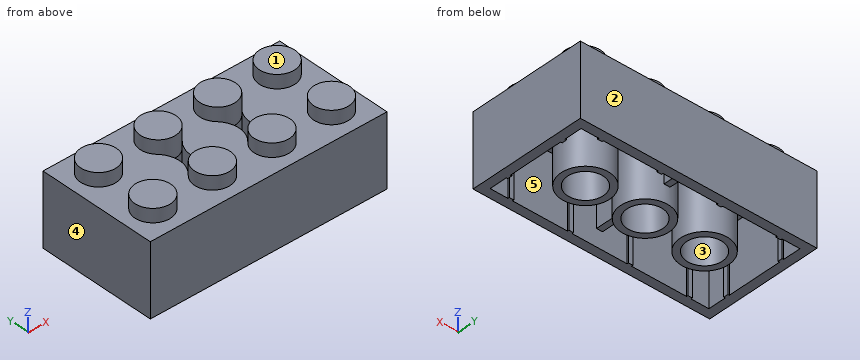
Autodesk Fusion 360 part; units mm, degrees
sketch "side" plane through (0, 0, 0) normal (1, 0, 0) x (0, 1, 0)
  line L0 (0, 0) -> (15.8, 0)
  line L1 (15.8, 0) -> (15.8, 9.6)
  line L2 (15.8, 9.6) -> (0, 9.6)
  line L3 (0, 9.6) -> (0, 0)
  dimension "d1" = 15.8
  dimension "d2" = 9.6
sketch "top" plane through (0, 0, 0) normal (0, 0, 1) x (1, 0, 0)
  line L0 (0, 0) -> (-31.8, 0)
  line L1 (-31.8, 0) -> (-31.8, 15.8)
  line L2 (-31.8, 15.8) -> (0, 15.8)
  line L3 (0, 15.8) -> (0, 0)
  circle A0 centre (-3.9, 11.9) radius 2.4
  line L4 (0, 15.8) -> (0, 0)
  circle A1 centre (-11.9, 11.9) radius 2.4
  circle A2 centre (-19.9, 11.9) radius 2.4
  circle A3 centre (-27.9, 11.9) radius 2.4
  circle A4 centre (-3.9, 3.9) radius 2.4
  circle A5 centre (-11.9, 3.9) radius 2.4
  circle A6 centre (-19.9, 3.9) radius 2.4
  circle A7 centre (-27.9, 3.9) radius 2.4
  circle A8 centre (-7.9, 7.9) radius 3.255
  circle A9 centre (-7.9, 7.9) radius 2.4
  circle A10 centre (-3.9, 11.9) radius 1.3
  circle A11 centre (-3.9, 3.9) radius 1.3
  circle A12 centre (-11.9, 11.9) radius 1.3
  circle A13 centre (-11.9, 3.9) radius 1.3
  circle A14 centre (-19.9, 11.9) radius 1.3
  circle A15 centre (-19.9, 3.9) radius 1.3
  circle A16 centre (-27.9, 11.9) radius 1.3
  circle A17 centre (-27.9, 3.9) radius 1.3
  circle A18 centre (-15.9, 7.9) radius 3.255
  circle A19 centre (-23.9, 7.9) radius 3.255
  circle A20 centre (-15.9, 7.9) radius 2.4
  circle A21 centre (-23.9, 7.9) radius 2.4
  line L5 (-30.6, 14.6) -> (-1.2, 14.6)
  line L6 (-1.2, 14.6) -> (-1.2, 1.2)
  line L7 (-1.2, 1.2) -> (-30.6, 1.2)
  line L8 (-30.6, 1.2) -> (-30.6, 14.6)
  line L9 (-15.9, 7.9) -> (-15.9, 14.6) construction
  line L10 (-15.9, 7.9) -> (-15.9, 1.2) construction
  line L11 (-16.3, 11.1303) -> (-16.3, 14.6)
  line L12 (-15.5, 11.1303) -> (-15.5, 14.6)
  line L13 (-15.5, 4.6697) -> (-15.5, 1.2)
  line L14 (-16.3, 4.6697) -> (-16.3, 1.2)
  line L15 (-28.2, 14.6) -> (-27.6, 14.6)
  line L16 (-27.6, 14.6) -> (-27.6, 14.4)
  line L17 (-27.6, 14.4) -> (-28.2, 14.4)
  line L18 (-28.2, 14.4) -> (-28.2, 14.6)
  line L19 (-20.2, 14.6) -> (-19.6, 14.6)
  line L20 (-19.6, 14.6) -> (-19.6, 14.4)
  line L21 (-19.6, 14.4) -> (-20.2, 14.4)
  line L22 (-20.2, 14.4) -> (-20.2, 14.6)
  line L23 (-12.2, 14.6) -> (-11.6, 14.6)
  line L24 (-11.6, 14.6) -> (-11.6, 14.4)
  line L25 (-11.6, 14.4) -> (-12.2, 14.4)
  line L26 (-12.2, 14.4) -> (-12.2, 14.6)
  line L27 (-4.2, 14.4) -> (-3.6, 14.4)
  line L28 (-3.6, 14.4) -> (-3.6, 14.6)
  line L29 (-3.6, 14.6) -> (-4.2, 14.6)
  line L30 (-4.2, 14.6) -> (-4.2, 14.4)
  line L31 (-1.4, 12.2) -> (-1.2, 12.2)
  line L32 (-1.2, 12.2) -> (-1.2, 11.6)
  line L33 (-1.2, 11.6) -> (-1.4, 11.6)
  line L34 (-1.4, 11.6) -> (-1.4, 12.2)
  line L35 (-1.4, 4.2) -> (-1.2, 4.2)
  line L36 (-1.2, 4.2) -> (-1.2, 3.6)
  line L37 (-1.2, 3.6) -> (-1.4, 3.6)
  line L38 (-1.4, 3.6) -> (-1.4, 4.2)
  line L39 (-4.2, 1.4) -> (-3.6, 1.4)
  line L40 (-3.6, 1.4) -> (-3.6, 1.2)
  line L41 (-3.6, 1.2) -> (-4.2, 1.2)
  line L42 (-4.2, 1.2) -> (-4.2, 1.4)
  line L43 (-11.6, 1.4) -> (-12.2, 1.4)
  line L44 (-12.2, 1.4) -> (-12.2, 1.2)
  line L45 (-12.2, 1.2) -> (-11.6, 1.2)
  line L46 (-11.6, 1.2) -> (-11.6, 1.4)
  line L47 (-19.6, 1.4) -> (-20.2, 1.4)
  line L48 (-20.2, 1.4) -> (-20.2, 1.2)
  line L49 (-20.2, 1.2) -> (-19.6, 1.2)
  line L50 (-19.6, 1.2) -> (-19.6, 1.4)
  line L51 (-27.6, 1.4) -> (-28.2, 1.4)
  line L52 (-28.2, 1.4) -> (-28.2, 1.2)
  line L53 (-28.2, 1.2) -> (-27.6, 1.2)
  line L54 (-27.6, 1.2) -> (-27.6, 1.4)
  line L55 (-30.4, 4.2) -> (-30.6, 4.2)
  line L56 (-30.6, 4.2) -> (-30.6, 3.6)
  line L57 (-30.6, 3.6) -> (-30.4, 3.6)
  line L58 (-30.4, 3.6) -> (-30.4, 4.2)
  line L59 (-30.4, 12.2) -> (-30.6, 12.2)
  line L60 (-30.6, 12.2) -> (-30.6, 11.6)
  line L61 (-30.6, 11.6) -> (-30.4, 11.6)
  line L62 (-30.4, 11.6) -> (-30.4, 12.2)
  dimension "d3" = 31.8
  dimension "d4" = 15.8
  dimension "d5" = 4.8
  dimension "d6" = 3.9
  dimension "d7" = 3.9
  dimension "d8" = 4.8
  dimension "d9" = 4.8
  dimension "d10" = 4.8
  dimension "d11" = 4.8
  dimension "d12" = 4.8
  dimension "d13" = 4.8
  dimension "d14" = 4.8
  dimension "d15" = 3.9
  dimension "d16" = 3.9
  dimension "d17" = 3.9
  dimension "d18" = 8
  dimension "d19" = 8
  dimension "d20" = 8
  dimension "d21" = 8
  dimension "d22" = 8
  dimension "d23" = 8
  dimension "d24" = 3.9
  dimension "d25" = 8
  dimension "d26" = 8
  dimension "d27" = 8
  dimension "d28" = 8
  dimension "d29" = 6.51
  dimension "d30" = 7.9
  dimension "d31" = 7.9
  dimension "d32" = 4.8
  dimension "d33" = 2.6
  dimension "d34" = 2.6
  dimension "d35" = 2.6
  dimension "d36" = 2.6
  dimension "d37" = 2.6
  dimension "d38" = 2.6
  dimension "d39" = 2.6
  dimension "d40" = 2.6
  dimension "d41" = 6.51
  dimension "d42" = 6.51
  dimension "d43" = 8
  dimension "d44" = 7.9
  dimension "d45" = 8
  dimension "d46" = 7.9
  dimension "d47" = 4.8
  dimension "d48" = 4.8
  dimension "d49" = 1.2
  dimension "d50" = 1.2
  dimension "d51" = 1.2
  dimension "d52" = 1.2
  dimension "d53" = 0.8
  dimension "d54" = 0.4
  dimension "d55" = 0.4
  dimension "d56" = 0.8
  dimension "d57" = 0.6
  dimension "d58" = 0.2
  dimension "d60" = 0.6
  dimension "d61" = 0.3
  dimension "d62" = 0.6
  dimension "d63" = 0.3
  dimension "d64" = 0.6
  dimension "d65" = 0.3
  dimension "d66" = 0.6
  dimension "d67" = 0.3
  dimension "d68" = 0.6
  dimension "d69" = 0.6
  dimension "d70" = 0.6
  dimension "d71" = 0.6
  dimension "d72" = 0.6
  dimension "d73" = 0.6
  dimension "d74" = 0.3
  dimension "d75" = 0.6
extrude "Extrude1" add sketch "top" along normal blind 9.6 contours L0 L1 L2 L3 L4 | L5 L23 L24 L25 L26 | L5 L19 L20 L21 L22 | L7 L43 L44 L45 L46 | L5 L27 L28 L29 L30 | L7 L47 L48 L49 L50 | L5 L15 L16 L17 L18 | L7 L39 L40 L41 L42 | L7 L51 L52 L53 L54 | L6 L31 L32 L33 L34 | L8 L59 L60 L61 L62 | L6 L35 L36 L37 L38 | L8 L55 L56 L57 L58 makes body 1
extrude "Extrude2" add sketch "top" along normal blind 9.6 and the other way blind -8.6 contours A0 | A4 | A1 A5 A8 A18 L5 L6 L7 L12 L13 L24 L25 L26 L27 L28 L30 L31 L33 L34 L35 L37 L38 L39 L40 L42 L43 L44 L46 | A8 | A1 | A18 | A5 | A18 L5 L11 L12 | A7 | A3 | A2 A6 A18 A19 L5 L7 L8 L11 L14 L16 L17 L18 L20 L21 L22 L47 L48 L50 L51 L52 L54 L55 L57 L58 L59 L61 L62 | A18 L7 L13 L14 | A2 | A19 | A6 | A9 | A20 | A21 bodies 1
extrude "Extrude3" add sketch "top" along normal blind 9.6 and the other way blind -11.4 contours A0 | A4 | A1 | A5 | A7 | A3 | A2 | A6 | A10 | A11 | A12 | A13 | A14 | A15 | A16 | A17 bodies 1
extrude "Extrude4" cut sketch "top" along normal blind 10.3 and the other way blind -9.6 contours A10 | A11 | A12 | A13 | A14 | A15 | A16 | A17 bodies 1
extrude "Extrude5" add sketch "top" along normal blind 8.6 contours A8 | A18 | A19 bodies 1
extrude "Extrude6" add sketch "top" along normal blind 8.6 and the other way blind -2.3 contours A18 L5 L11 L12 | A18 L7 L13 L14 bodies 1
copy_body "Body->Comp1" bodies 1 removing the originals makes body 2 in component "Piesa Lego 4x2"
component "Piesa Lego 4x2" placed x (1, 0, 0) y (0, 1, 0) z (0, 0, 1) at (0, 0, 0)
equation "d84 = -9.6 mm - 1.8 mm"
equation "d86 = 8.60 mm + 1.7 mm"
For this review, take the finished solid that the model builds, in its own axes (mm). Face numbers are marked on the shaded views. A direction names the side the tool comes from. Round coordinates to 2 decimals unless told otherwise and drop trailing zeros. Order: outer loops, then holes, each group sorted by start corner. A loop starts at its lowest first (then second) coordinate and runs counter-clockwise, first axis right, second up. Notation, with made-up numbers: (81, 30) -> (124, 30) arc R9 cw to (124, 43) -> close; hole circle Ø6 at (49, 46.5). An arc over 180 degrees is marked (long way). Use a Markdown table: item, result.
Item 1: Draft analysis for pull direction Y (two halves, no side actions). For the marked faces 1, 2 and 3, state which applies: +Y half, -Y half, draft (parallel to the pull), parting line (faces both ways), or undercut.
Resolved:
| item | result |
|---|---|
| face 1 | draft |
| face 2 | +Y half |
| face 3 | undercut |
Item 2: For pin 1 (4 mm diameter, centred on x = -3.9, y = 11.9, fed in from -Z), flat-tipped, find the tip position at first contact; note if it passes through.
Resolved:
| item | result |
|---|---|
| pin 1 | stops at z = 8.6 |
Item 3: Take a section at D-D (z = 4.5). State how many separate pieces and enclosed holes the cut face has, plus the area to 3 significant figures.
Resolved:
| item | result |
|---|---|
| separate pieces | 3 |
| enclosed holes | 5 |
| area | 161 mm² |
Item 4: For line 1 along X through (y, z) = (1.5, 7.25); line 2 along Y through (x, z) = (-23.9, 2.5) (3 decimals); line 3 along X through (y, z) = (4, 6.25), list the stretches that pass through material, from the lowest coordinate up. Write a range as [from, to].
Resolved:
| item | result |
|---|---|
| line 1 | x = [-31.8, -30.6], [-16.3, -15.5], [-1.2, 0] |
| line 2 | y = [0, 1.2], [4.645, 5.5], [10.3, 11.155], [14.6, 15.8] |
| line 3 | x = [-31.8, -30.4], [-16.3, -15.5], [-1.4, 0] |
Item 5: Take a section at A-A (x = -11.9). State the section outline as (y, z) points, plus the area to 3 significant figures.
Resolved:
| item | result |
|---|---|
| outline | (0, 0) -> (1.4, 0) -> (1.4, 8.6) -> (2.6, 8.6) -> (2.6, 10.3) -> (5.2, 10.3) -> (5.2, 8.6) -> (6.3, 8.6) -> (6.3, 11.4) -> (1.5, 11.4) -> (1.5, 9.6) -> (0, 9.6) -> close; (9.5, 8.6) -> (10.6, 8.6) -> (10.6, 10.3) -> (13.2, 10.3) -> (13.2, 8.6) -> (14.4, 8.6) -> (14.4, 0) -> (15.8, 0) -> (15.8, 9.6) -> (14.3, 9.6) -> (14.3, 11.4) -> (9.5, 11.4) -> close |
| area | 45.1 mm² |
Item 6: Take a section at B-B (x = -27.9). State the section outline as (y, z) points, plus the area to 3 significant figures.
Resolved:
| item | result |
|---|---|
| outline | (0, 0) -> (1.4, 0) -> (1.4, 8.6) -> (2.6, 8.6) -> (2.6, 10.3) -> (5.2, 10.3) -> (5.2, 8.6) -> (10.6, 8.6) -> (10.6, 10.3) -> (13.2, 10.3) -> (13.2, 8.6) -> (14.4, 8.6) -> (14.4, 0) -> (15.8, 0) -> (15.8, 9.6) -> (14.3, 9.6) -> (14.3, 11.4) -> (9.5, 11.4) -> (9.5, 9.6) -> (6.3, 9.6) -> (6.3, 11.4) -> (1.5, 11.4) -> (1.5, 9.6) -> (0, 9.6) -> close |
| area | 48.3 mm² |
Item 7: Machinability: for the marked faces 4 and 5, which of the approach directions +Z, -Z, +X, -X, +Y, -Y give a long, thin tool a straight path to every point of the face, cutting with its end or side? Answer none if there is none.
Resolved:
| item | result |
|---|---|
| face 4 | +Z, -Z, -X, +Y, -Y |
| face 5 | -Z |
